Can you work these out from the model? Positions are in its coordinate system, mm. Face numbers are marked on the shaded views. A direction names the side the tool comes from. Coordinates: 2 decimals unless noted, no trailing zeros. Order: outer loops, then holes, each group sorted by start corner. A loop starts at its lowest first (then second) coordinate and runs counter-clockwise, first axis right, second up.
```python
from build123d import *

# Parameters (mm, degrees)
SKETCH1_R           = 6.223
SKETCH1_R_2         = 4.7625
EXTRUDE1_DEPTH      = 0.508
EXTRUDE2_DEPTH      = 3.2258
EXTRUDE2_DEPTH_BACK = 3.2258
SKETCH3_W           = 0.901351443
SKETCH3_H           = 6.4516
EXTRUDE3_DEPTH      = 0.508
FILLET1_R           = 1.27


with BuildPart() as part:
    # Sketch1 → Extrude1 (new body)
    with BuildSketch(Plane.XY):
        Circle(SKETCH1_R)
        Circle(SKETCH1_R_2, mode=Mode.SUBTRACT)
    extrude(amount=EXTRUDE1_DEPTH)



with BuildPart() as body_2:
    # Sketch2 → Extrude2 (new, two sides: drawn at the far end of the back side and taken through both)
    with BuildSketch(Plane(origin=(0, 0, 0), x_dir=(1, 0, 0), z_dir=(0, 1, 0)).offset(-EXTRUDE2_DEPTH_BACK)):
        with BuildLine():
            Line((-6.223, 0), (-7.493, 0))
            ThreePointArc((-7.493, 0), (-8.391025612, -0.371974388), (-8.763, -1.27))
            Line((-8.763, -1.27), (-8.763, -17.907))
            ThreePointArc((-8.763, -17.907), (-6.08420147, -21.450454304), (-1.94460825, -19.839306284))
            Line((-1.94460825, -19.839306284), (-0.512193665, -17.537255749))
            ThreePointArc((-0.512193665, -17.537255749), (-0.292109819, -16.558154348), (-0.728518239, -15.654481761))
            Line((-0.728518239, -15.654481761), (-3.048, -13.335))
            Line((-3.048, -13.335), (-3.407210245, -13.694210245))
            Line((-3.407210245, -13.694210245), (-1.087728484, -16.013692006))
            ThreePointArc((-1.087728484, -16.013692006), (-0.796789537, -16.616140397), (-0.943512101, -17.268874664))
            Line((-0.943512101, -17.268874664), (-2.376524764, -19.571886378))
            ThreePointArc((-2.376524764, -19.571886378), (-5.945185277, -20.961845239), (-8.255, -17.907))
            Line((-8.255, -17.907), (-8.255, -1.27))
            ThreePointArc((-8.255, -1.27), (-8.031815367, -0.731184633), (-7.493, -0.508))
            Line((-7.493, -0.508), (-6.223, -0.508))
            Line((-6.223, -0.508), (-6.223, 0))
        make_face()
    extrude(amount=EXTRUDE2_DEPTH + EXTRUDE2_DEPTH_BACK)


with BuildPart() as part_1:
    add(part.part)

    add(body_2.part)  # Extrude3 merges body 2
    # Sketch3 → Extrude3 (add)
    with BuildSketch(Plane(origin=(0, 0, 0), x_dir=(-1, 0, 0), z_dir=(0, 0, -1))):
        with Locations((5.772324279, 0)):
            Rectangle(SKETCH3_W, SKETCH3_H)
    extrude(amount=-EXTRUDE3_DEPTH)

    # Fillet1
    fillet1_edges = [part_1.edges().sort_by_distance(p)[0] for p in [
        (-3.227605122, -3.2258, 13.514605122),
        (-3.227605122, 3.2258, 13.514605122),
    ]]
    fillet(fillet1_edges, radius=FILLET1_R)


solid = part_1.part
```
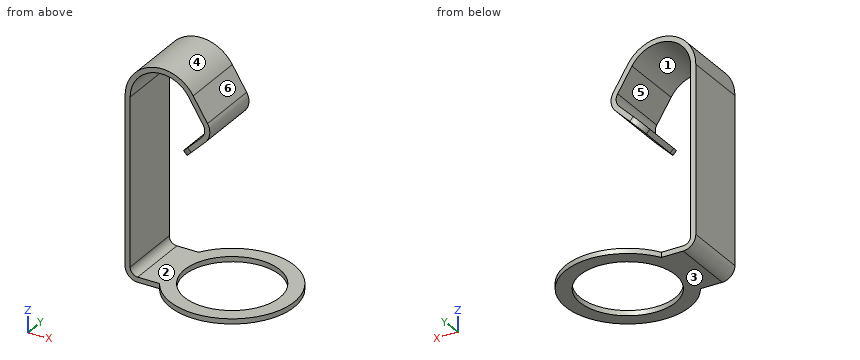
1. Imagine slicing it at C-C on x = -4.5. Please give me the cut outline in (y, z), then the cut area to 3 significant figures.
Completed:
outline: (-4.3, 0) - (-1.56, 0) - (-1.56, 0.51) - (-4.3, 0.51) - close; (-3.23, 21.03) - (3.23, 21.03) - (3.23, 21.54) - (-3.23, 21.54) - close; (1.56, 0) - (4.3, 0) - (4.3, 0.51) - (1.56, 0.51) - close
area: 6.11 mm2
2. Thinking about a two-plate mould opening in X: for the marked faces 4, 5 and 6, which applies, pulls with the +X half, pulls with the -X half, needs draft (parallel to the pull), parting line crosses it, or undercut?
Completed:
face 4: parting line crosses it
face 5: undercut
face 6: pulls with the +X half
3. I'm going to push flat-ended pins straight in: pin 1 (5 mm diameter, centred on x = 1.5, y = -1, fed in from -Z); pin 2 (3 mm diameter, centred on y = 0, z = 6.5, fed in from +X) (3 decimals). Where does each tip first touch, or does it pass through?
Completed:
pin 1: stops at z = 15.38
pin 2: stops at x = -8.255
4. Imagine slicing it at D-D on y = -4. Please give me the cut outline in (x, z).
Completed:
outline: (-4.77, 0) - (-2.58, 0) - (-2.58, 0.51) - (-4.77, 0.51) - close; (2.58, 0) - (4.77, 0) - (4.77, 0.51) - (2.58, 0.51) - close
5. On a 3-axis mill with a long thin cutter (end or side, diameter ignored), from which of +Z, -Z, +X, -X, +Y, -Y can I reach the whole of each face in a straight line? I mean the marked faces 1, 2 and 3. Say none if no direction works.
Completed:
face 1: +Y, -Y
face 2: +X, +Y, -Y
face 3: -Z, +X, -X, +Y, -Y
6. Imagine slicing it at B-B on x = 0. Please give me the cut outline in (y, z), then the cut area to 3 significant figures.
Completed:
outline: (-6.22, 0) - (-4.76, 0) - (-4.76, 0.51) - (-6.22, 0.51) - close; (4.76, 0) - (6.22, 0) - (6.22, 0.51) - (4.76, 0.51) - close
area: 1.48 mm2
7. Please list where these lines run through material, in increasing order: probe 1 along Y at (x, z) = (0, 0.35); probe 2 along Z at (x, y) = (-5.25, 1); probe 3 along Z at (x, y) = (-2.25, 5.5).
Completed:
probe 1: y = -6.22 to -4.76, 4.76 to 6.22
probe 2: z = 0 to 0.51, 21.08 to 21.59
probe 3: z = 0 to 0.51
